```python
from build123d import *

# Parameters (mm, degrees)
SKETCH1_W           = 10.922
SKETCH1_H           = 7.874
BOSS_EXTRUDE1_DEPTH = 9.906
SKETCH2_R           = 2.286
BOSS_EXTRUDE2_DEPTH = 5.334
SKETCH3_R           = 2.4892
BOSS_EXTRUDE3_DEPTH = 3.556
SKETCH4_R           = 1.524
BOSS_EXTRUDE4_DEPTH = 1.905
SKETCH5_R           = 1
CUT_EXTRUDE1_DEPTH  = 3.81
SKETCH7_R           = 0.889
CUT_EXTRUDE2_DEPTH  = 3.81
SKETCH8_W           = 1.221154325
SKETCH8_H           = 1.27
BOSS_EXTRUDE5_DEPTH = 0.254


with BuildPart() as part:
    # Sketch1 → Boss-Extrude1 (new body)
    with BuildSketch(Plane.XY):
        Rectangle(SKETCH1_W, SKETCH1_H)
    extrude(amount=BOSS_EXTRUDE1_DEPTH)

    # Sketch2 → Boss-Extrude2 (add)
    with BuildSketch(Plane(origin=(5.461, 0, 0), x_dir=(0, 0, -1), z_dir=(1, 0, 0))):
        with Locations((-4.953, 0)):
            Circle(SKETCH2_R)
    extrude(amount=BOSS_EXTRUDE2_DEPTH)

    # Sketch3 → Boss-Extrude3 (add)
    with BuildSketch(Plane(origin=(10.795, 0, 0), x_dir=(0, 0, -1), z_dir=(1, 0, 0))):
        with Locations((-4.953, 0)):
            Circle(SKETCH3_R)
    extrude(amount=BOSS_EXTRUDE3_DEPTH)

    # Sketch4 → Boss-Extrude4 (add)
    with BuildSketch(Plane.ZY.offset(5.461)):
        with Locations((4.953, 0)):
            Circle(SKETCH4_R)
    extrude(amount=BOSS_EXTRUDE4_DEPTH)

    # Sketch5 → Cut-Extrude1 (cut)
    with BuildSketch(Plane.XY.offset(9.906)):
        with Locations((2.197310811, -1.890493537)):
            Circle(SKETCH5_R)
        with Locations((-2.781089189, 2.300506463)):
            Circle(SKETCH5_R)
    extrude(amount=-CUT_EXTRUDE1_DEPTH, mode=Mode.SUBTRACT)

    # Sketch7 → Cut-Extrude2 (cut)
    with BuildSketch(Plane(origin=(0, -2.4892, 0), x_dir=(1, 0, 0), z_dir=(0, 1, 0))):
        with Locations((12.573, -4.953)):
            Circle(SKETCH7_R)
    extrude(amount=CUT_EXTRUDE2_DEPTH, mode=Mode.SUBTRACT)

    # Sketch8 → Boss-Extrude5 (add)
    with BuildSketch(Plane.XY):
        with Locations((-6.071577163, 0)):
            Rectangle(SKETCH8_W, SKETCH8_H)
    extrude(amount=BOSS_EXTRUDE5_DEPTH)


solid = part.part
```
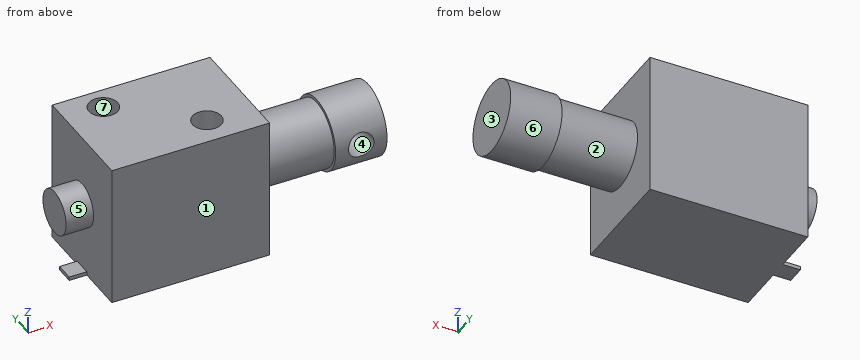
The listing builds one solid part. Answer for the finished solid, in the listing's coordinates (mm). Face numbers are marked on the shaded views. A direction names the side the tool comes from. Round coordinates to 2 decimals unless told otherwise and drop trailing zeros. Order: outer loops, then holes, each group sorted by start corner. A loop starts at its lowest first (then second) coordinate and runs counter-clockwise, first axis right, second up. Notation, with made-up numbers: (18, 26) -> (65, 26) arc R27 cw to (65, 64) -> close; hole circle Ø4 at (11.5, 19.25). An arc over 180 degrees is marked (long way). Answer as CSV lines item,"result".
Q1. For a pull along X with two mould halves and no side action, classify the marked faces 1, 2 and 3 as +X half, -X half, draft (parallel to the pull), parting line (faces both ways), or undercut.
Computed values:
face 1,"draft"
face 2,"undercut"
face 3,"+X half"
Q2. Which of the six approach directions +Z, -Z, +X, -X, +Y, -Y give full straight-line access (tool end or side, diameter ignored) to the marked faces 4, 5, 6 and 7?
Computed values:
face 4,"-Y"
face 5,"-X"
face 6,"+X"
face 7,"+Z"
Q3. A cutting plane is placed at D-D on z = 4.5. Determine the outline of the cut face in (x, y) (3 decimals), plus the area to 3 significant figures.
Computed values:
outline,"(-7.366, -1.455) -> (-5.461, -1.455) -> (-5.461, -3.937) -> (5.461, -3.937) -> (5.461, -2.241) -> (10.795, -2.241) -> (10.795, -2.448) -> (11.808, -2.448) -> (11.808, 1.321) -> (13.338, 1.321) -> (13.338, -2.448) -> (14.351, -2.448) -> (14.351, 2.448) -> (10.795, 2.448) -> (10.795, 2.241) -> (5.461, 2.241) -> (5.461, 3.937) -> (-5.461, 3.937) -> (-5.461, 1.455) -> (-7.366, 1.455) -> close"
area,"127 mm^2"
Q4. A cutting plane is placed at A-A on y = 0. Determine the outline of the cut face in (x, z) (3 decimals).
Computed values:
outline,"(-7.366, 3.429) -> (-5.461, 3.429) -> (-5.461, 0.254) -> (-6.682, 0.254) -> (-6.682, 0) -> (5.461, 0) -> (5.461, 2.667) -> (10.795, 2.667) -> (10.795, 2.464) -> (14.351, 2.464) -> (14.351, 7.442) -> (10.795, 7.442) -> (10.795, 7.239) -> (5.461, 7.239) -> (5.461, 9.906) -> (-5.461, 9.906) -> (-5.461, 6.477) -> (-7.366, 6.477) -> close; hole circle Ø1.778 at (12.573, 4.953)"
Q5. A cutting plane is placed at B-B on z = 8. Determine the outline of the cut face in (x, y).
Computed values:
outline,"(-5.46, -3.94) -> (5.46, -3.94) -> (5.46, 3.94) -> (-5.46, 3.94) -> close; hole circle Ø2 at (-2.78, 2.3); hole circle Ø2 at (2.2, -1.89)"
Q6. Given pin 1 (2 mm diameter, centred on x = 9, z = 7.5, fed in from +Y); pin 2 (1 mm diameter, centred on x = -3, y = 2.5, fed in from +Z); pin 3 (3 mm diameter, centred on y = 3, z = 8, fed in from +X), each flat-ended and moving along its own axis, determine where each tip first touches the part or whether it passes through.
Computed values:
pin 1,"stops at y = 1.68"
pin 2,"stops at z = 6.1"
pin 3,"stops at x = 5.46"
Q7. Consider line 1 (X direction, y = -0.5, z = 5); line 2 (X direction, y = -1, z = 3); line 3 (X direction, y = -2.75, z = 7). Determine where each line is inside the solid, lowest interval first. Write a range as from..to.
Computed values:
line 1,"x = -7.37..11.69, 13.46..14.35"
line 2,"x = -5.46..14.35"
line 3,"x = -5.46..1.69, 2.71..5.46"
Q8. A cutting plane is placed at C-C on x = -2.25. Determine the outline of the cut face in (y, z), plus the area to 3 significant figures.
Computed values:
outline,"(-3.94, 0) -> (3.94, 0) -> (3.94, 9.91) -> (3.15, 9.91) -> (3.15, 6.1) -> (1.45, 6.1) -> (1.45, 9.91) -> (-3.94, 9.91) -> close"
area,"71.5 mm^2"
